Input: part model. Units: mm. Frame: model coordinates. A direction names the side the tool comes from. Give positions to 0.01 mm unless a question says otherwise; leave off trailing zeros. Loops run counter-clockwise (first coordinate to the right, second up) from the corner with the lowest first, then second, coordinate; pieces in that order, holes last. Notation, with made-up numbers: (75, 32) - (86, 32) arc R18 cw to (86, 42) - close; hole circle Ø10 at (-27, 45). An arc over 180 degrees is marked (long way). Answer as a JSON object with one key per item and string values. Group by question number.
(1) Section query C-C (x = 9). Return loops of the section in (y, z).
(2) Section query B-B (y = 55.25). Return loops of the section in (x, z).
(3) Material intervals for L1, parallel to Z at x = -7, y = 55; L2, parallel to Y at x = 9, z = -1; L3, parallel to X at y = 54, z = 34.5, sorted ascending.
(4) Access query for faces 4 (the flat face through (-21, 18.5, 25)), 5 (the cylindrical face through (-6.9, 16.36, 25.35)), 6 (the flat face through (-21, 64, 25)), 7 (the cylindrical face through (0.035, 67.723, -1.634)). Directions: +Z, -Z, +X, -X, +Y, -Y. A direction counts if a zero-diameter tool reaches every point of the face in a straight line with its end or side. Return the directions, or none.
(5) Section query D-D (z = 14). Count the separate pieces of the cut face and the enclosed holes in it, plus the area to 3 significant figures.
(6) Pin query (flat end, axial travel): P1, Ø19, axis at x = -20, z = 29.5, coming from the +Y side; P2, Ø4.5, axis at x = 9, y = 43, coming from the +Z side; P3, Ø5, axis at x = 9, y = 29, coming from the -Z side; P4, Ø4.5, axis at y = 24.25, z = 45, coming from the +X side. Return the tip coordinate at first contact, or that it passes through.
(7) Mould query, pull axis Z, two halves, no side actions, for faces 1 (the cylindrical face through (27.923, 41.226, -1.479)), 2 (the cylindrical face through (-7.479, 56.867, 44.33)), 3 (the flat face through (0, 37, -3)). Classes: +Z half, -Z half, draft (parallel to the pull), parting line (faces both ways), or undercut.
```python
from build123d import *

# Parameters (mm, degrees)
F0_W      = 68
F0_H      = 72
F0_R      = 2
F1_DEPTH  = 3
F3_DEPTH  = 50
F4_SIZE   = 10
F6_R      = 1.75
F6_R_2    = 12
F7_DEPTH  = 25
F8_R      = 5
F9_R      = 1.49999
F10_R     = 3
F11_R     = 0.5
F13_R     = 20
F13_R_2   = 1.75
F14_DEPTH = 2.5


# Not quite as in the source:
# - a fillet or chamfer is up to 0.001 mm smaller than in the source, because OpenCascade refuses the exact size


with BuildPart() as f1:
    # F0 (on Top) → F1 (new body)
    with BuildSketch(Plane.XY):
        with Locations((0, 36)):
            Rectangle(F0_W, F0_H)
        with Locations((-9, 5)):
            Circle(F0_R, mode=Mode.SUBTRACT)
        with Locations((-9, 29)):
            Circle(F0_R, mode=Mode.SUBTRACT)
        with Locations((9, 5)):
            Circle(F0_R, mode=Mode.SUBTRACT)
        with Locations((9, 29)):
            Circle(F0_R, mode=Mode.SUBTRACT)
        with Locations((-27, 43)):
            Circle(F0_R, mode=Mode.SUBTRACT)
        with Locations((-9, 43)):
            Circle(F0_R, mode=Mode.SUBTRACT)
        with Locations((-27, 67)):
            Circle(F0_R, mode=Mode.SUBTRACT)
        with Locations((-9, 67)):
            Circle(F0_R, mode=Mode.SUBTRACT)
        with Locations((9, 43)):
            Circle(F0_R, mode=Mode.SUBTRACT)
        with Locations((27, 43)):
            Circle(F0_R, mode=Mode.SUBTRACT)
        with Locations((9, 67)):
            Circle(F0_R, mode=Mode.SUBTRACT)
        with Locations((27, 67)):
            Circle(F0_R, mode=Mode.SUBTRACT)
        with Locations((-9, 43)):
            Circle(F0_R)
        with Locations((-9, 29)):
            Circle(F0_R)
    extrude(amount=-F1_DEPTH)

    # F2 (on Top) → F3 (join)
    with BuildSketch(Plane.XY):
        Polygon((-6, 64), (-34, 64), (-34, 61), (-9, 61), (-9, 18.5), (-34, 18.5), (-34, 15.5), (-6, 15.5), align=None)
    extrude(amount=F3_DEPTH)

    # F4
    f4_edges = [f1.edges().sort_by_distance(p)[0] for p in [
        (-34, 62.5, 50),
        (-34, 17, 50),
    ]]
    chamfer(f4_edges, length=F4_SIZE)

    # F6 (on face) → F7 (cut)
    with BuildSketch(Plane.YZ.offset(-6)):
        with Locations((55.25, 45)):
            Circle(F6_R)
        with Locations((39.75, 29.5)):
            Circle(F6_R_2)
        with Locations((55.25, 14)):
            Circle(F6_R)
        with Locations((24.25, 45)):
            Circle(F6_R)
        with Locations((24.25, 14)):
            Circle(F6_R)
    extrude(amount=-F7_DEPTH, mode=Mode.SUBTRACT)

    # F8
    f8_edges = [f1.edges().sort_by_distance(p)[0] for p in [
        (-34, 72, -1.5),
        (34, 72, -1.5),
        (34, 0, -1.5),
        (-34, 0, -1.5),
        (-34, 17, 40),
        (-34, 62.5, 40),
    ]]
    fillet(f8_edges, radius=F8_R)

    # F9 (radius 1.5 in the source; OpenCascade refuses exactly that, so slightly less here)
    f9_edges = [f1.edges().sort_by_distance(p)[0] for p in [
        (-34, 64, 18.964466),
        (-34, 61, 18.964466),
        (-28.267767, 15.5, 45.732233),
        (-28.267767, 18.5, 45.732233),
        (-33.619398, 15.5, 39.842349),
        (-34, 15.5, 18.964466),
        (-34, 18.5, 18.964466),
        (-33.619398, 18.5, 39.842349),
        (-33.619398, 64, 39.842349),
        (-33.619398, 61, 39.842349),
        (-28.267767, 61, 45.732233),
        (-28.267767, 64, 45.732233),
    ]]
    fillet(f9_edges, radius=F9_R)

    # F10
    f10_edges = [f1.edges().sort_by_distance(p)[0] for p in [
        (-6, 15.5, 25),
        (-6, 64, 25),
    ]]
    fillet(f10_edges, radius=F10_R)

    # F11
    f11_edges = [f1.edges().sort_by_distance(p)[0] for p in [
        (-9, 18.5, 25),
        (-9, 61, 25),
    ]]
    fillet(f11_edges, radius=F11_R)

    # F13 (on offset) → F14 (cut, symmetric)
    with BuildSketch(Plane.YZ):
        with Locations((55.25, 14)):
            Circle(F13_R)
        with Locations((55.25, 14)):
            Circle(F13_R_2, mode=Mode.SUBTRACT)
    extrude(amount=F14_DEPTH, both=True, mode=Mode.SUBTRACT)


solid = f1.part
```
Recorded:
{
 "1": {"outline": "(0, -3) - (3, -3) - (3, 0) - (0, 0) - close; (7, -3) - (27, -3) - (27, 0) - (7, 0) - close; (31, -3) - (41, -3) - (41, 0) - (31, 0) - close; (45, -3) - (65, -3) - (65, 0) - (45, 0) - close; (69, -3) - (72, -3) - (72, 0) - (69, 0) - close"},
 "2": {"outline": "(-34, -3) - (-2.5, -3) - (-2.5, 0) - (-6, 0) - (-6, 12.25) - (-9, 12.25) - (-9, 0) - (-34, 0) - close; (-9, 15.75) - (-6, 15.75) - (-6, 43.25) - (-9, 43.25) - close; (-9, 46.75) - (-6, 46.75) - (-6, 50) - (-9, 50) - close; (2.5, -3) - (34, -3) - (34, 0) - (2.5, 0) - close"},
 "3": {"L1": "z = -3 to 12.27, 15.73 to 43.27, 46.73 to 50", "L2": "y = 0 to 3, 7 to 27, 31 to 41, 45 to 65, 69 to 72", "L3": "x = -9 to -6"},
 "4": {"face 4": "+Z, -X", "face 5": "+Z, +X, -Y", "face 6": "+Z, +X, -X, +Y", "face 7": "+Z"},
 "5": {"separate pieces": "3", "enclosed holes": "0", "area": "269 mm^2"},
 "6": {"P1": "stops at y = 64", "P2": "stops at z = 0", "P3": "stops at z = -3", "P4": "stops at x = -6"},
 "7": {"face 1": "draft", "face 2": "undercut", "face 3": "-Z half"}
}
